from build123d import *

# Parameters (mm, degrees)
SKETCH_W        = 20
SKETCH_H        = 20
PAD_DEPTH       = 300
SKETCH001_R     = 2.5
POCKET_DEPTH    = 300.001
POCKET001_DEPTH = 300.001
SKETCH003_W     = 20
SKETCH003_H     = 20
POCKET002_DEPTH = 100


with BuildPart() as part:
    # Sketch → Pad (new body)
    with BuildSketch(Plane.XY):
        Rectangle(SKETCH_W, SKETCH_H)
    extrude(amount=PAD_DEPTH)

    # Sketch001 (on Face6 of Pad) → Pocket (cut, through all)
    with BuildSketch(Plane.XY.offset(300)):
        Circle(SKETCH001_R)
        Polygon((-3.1, 10), (3.1, 10), (3.1, 8), (6.232233, 8), (2.132233, 3.9), (-2.132233, 3.9), (-6.232233, 8), (-3.1, 8), align=None)
        Polygon((-3.1, -8), (-6.232233, -8), (-2.132233, -3.9), (2.132233, -3.9), (6.232233, -8), (3.1, -8), (3.1, -10), (-3.1, -10), align=None)
    extrude(amount=-POCKET_DEPTH, mode=Mode.SUBTRACT)

    # Sketch002 (on Face2 of Pocket) → Pocket001 (cut, through all)
    with BuildSketch(Plane(origin=(0, 0, 0), x_dir=(1, 0, 0), z_dir=(0, 0, -1))):
        Polygon((-10, -3.1), (-8, -3.1), (-8, -6.232233), (-3.9, -2.132233), (-3.9, 2.132233), (-8, 6.232233), (-8, 3.1), (-10, 3.1), align=None)
        Polygon((3.9, -2.132233), (3.9, 2.132233), (8, 6.232233), (8, 3.1), (10, 3.1), (10, -3.1), (8, -3.1), (8, -6.232233), align=None)
    extrude(amount=-POCKET001_DEPTH, mode=Mode.SUBTRACT)

    # Sketch003 (on Face4 of Clone) → Pocket002 (cut)
    with BuildSketch(Plane.XY.offset(300)):
        Rectangle(SKETCH003_W, SKETCH003_H)
    extrude(amount=-POCKET002_DEPTH, mode=Mode.SUBTRACT)


solid = part.part
Input: part model. Units: mm. Frame: model coordinates. A direction names the side the tool comes from. Coordinates: 2 decimals unless noted, no trailing zeros. Loops run counter-clockwise (first coordinate to the right, second up) from the corner with the lowest first, then second, coordinate; pieces in that order, holes last.
Q1. Material intervals for line 1 (Y direction, x = 0, z = 76); line 2 (X direction, y = 4.5, z = 71.5); line 3 (X direction, y = -4.25, z = 141.5), sorted ascending.
Q2. Contact query for flat-ended pins moving along their axis: pin 1 (3.5 mm diameter, centred on y = 0, z = 140.5, fed in from -X); pin 2 (1.3 mm diameter, centred on x = 0.5, z = 99.5, fed in from -Y); pin 3 (5 mm diameter, centred on x = -0.5, z = 167, fed in from -Y). Output: stop coordinate, or through.
Q3. Draft query along Y for faces 3 (the face through (-7, 10, 99)), 4 (the face through (-7, -10, 99)), 5 (the face through (4.21, 5.98, 101.4)), 6 (the face through (2, 2, 200)). Return one class per face: +Y half, -Y half, draft (parallel to the pull), parting line (faces both ways), or undercut.
Q4. Cut plane A-A (y = 0). Output: boundary loops of the cut face in (x, z), then the cut area to 3 significant figures.
Q5. Set-up query: faces 1 (the face through (-10, -7, 99)), 2 (the face through (-3.9, 0, 99)). Return all of +Z, -Z, +X, -X, +Y, -Y with unobstructed straight access to the full face (end or side cutting, diameter ignored); none if empty.
Working result:
1. line 1: y = -3.9 to -2.5, 2.5 to 3.9
1. line 2: x = -10 to -8, -6.27 to -2.73, 2.73 to 6.27, 8 to 10
1. line 3: x = -10 to -8, -6.02 to -2.48, 2.48 to 6.02, 8 to 10
2. pin 1: stops at x = -3.9
2. pin 2: stops at y = -3.9
2. pin 3: stops at y = -4.77
3. face 3: +Y half
3. face 4: -Y half
3. face 5: undercut
3. face 6: draft
4. outline: (-3.9, 0) - (-2.5, 0) - (-2.5, 200) - (-3.9, 200) - close; (2.5, 0) - (3.9, 0) - (3.9, 200) - (2.5, 200) - close
4. area: 560 mm2
5. face 1: +Z, -Z, -X, +Y, -Y
5. face 2: +Z, -Z, -X
